Verification items for the finished model (mm, model axes). Face numbers are marked on the shaded views. A direction names the side the tool comes from. Coordinates: 2 decimals unless noted, no trailing zeros. Write each loop counter-clockwise with the first axis right and the second up, starting at its lowest first coordinate (ties: lowest second). Pieces come first, ordered by that corner, then holes. Notation, with made-up numbers: M -14.75,83 L -1.75,83 A27 cw -1.75,121 Z; hole C 47,84 d11. An arc over 180 degrees is marked long. One line per item, written item: value.
```python
from build123d import *

# Parameters (mm, degrees)
BOSS_EXTRUDE1_DEPTH = 70.612
SKETCH2_R           = 2.2
CUT_EXTRUDE1_DEPTH  = 83.799422419
SKETCH3_W           = 8.255
SKETCH3_H           = 31.401404102
CUT_EXTRUDE2_DEPTH  = 83.799422419
BOSS_EXTRUDE3_DEPTH = 2.54
CUT_EXTRUDE6_DEPTH  = 2.54
SKETCH9_W           = 51.816
SKETCH9_H           = 2.54
CUT_EXTRUDE7_DEPTH  = 2.54
FILLET1_R           = 1.27
FILLET2_R           = 1.27
SKETCH11_W          = 16.51
SKETCH11_H          = 8.89
CUT_EXTRUDE8_DEPTH  = 2.54


with BuildPart() as part:
    # Sketch1 → Boss-Extrude1 (new body)
    with BuildSketch(Plane.XY):
        Polygon((25.908, 25.4), (-25.908, 25.4), (-25.908, 0), (-36.703, 0), (-36.703, 5.08), (-28.448, 5.08), (-28.448, 27.94), (28.448, 27.94), (28.448, 5.08), (36.703, 5.08), (36.703, 0), (25.908, 0), align=None)
    extrude(amount=BOSS_EXTRUDE1_DEPTH)

    # Sketch2 → Cut-Extrude1 (cut, through all)
    with BuildSketch(Plane(origin=(0, 5.08, 0), x_dir=(1, 0, 0), z_dir=(0, 1, 0))):
        with Locations(Location((-32.5755, -6.35, 0), (0, 0, 270))):
            Circle(SKETCH2_R)
        with Locations(Location((-32.5755, -29.21, 0), (0, 0, 270))):
            Circle(SKETCH2_R)
    cut_extrude1 = extrude(amount=-CUT_EXTRUDE1_DEPTH, mode=Mode.SUBTRACT)

    # Mirror1: Cut-Extrude1 across plane
    add(cut_extrude1.mirror(Plane(origin=(0, 0, 0), x_dir=(0, 0, 1), z_dir=(1, 0, 0))), mode=Mode.SUBTRACT)

    # Sketch3 → Cut-Extrude2 (cut, through all)
    with BuildSketch(Plane(origin=(0, 5.08, 0), x_dir=(1, 0, 0), z_dir=(0, 1, 0))):
        with Locations((-32.5755, -54.911297949)):
            Rectangle(SKETCH3_W, SKETCH3_H)
        with Locations((32.5755, -54.911297949)):
            Rectangle(SKETCH3_W, SKETCH3_H)
    extrude(amount=-CUT_EXTRUDE2_DEPTH, mode=Mode.SUBTRACT)

    # Sketch6 → Boss-Extrude3 (add)
    with BuildSketch(Plane(origin=(0, 0, 0), x_dir=(-1, 0, 0), z_dir=(0, 0, -1))):
        Polygon((-25.908, 0), (25.908, 0), (36.703, 0), (36.703, 5.08), (28.448, 5.08), (28.448, 27.94), (-28.448, 27.94), (-28.448, 5.08), (-36.703, 5.08), (-36.703, 0), align=None)
    extrude(amount=-BOSS_EXTRUDE3_DEPTH)

    # Sketch8 → Cut-Extrude6 (cut)
    with BuildSketch(Plane(origin=(0, 0, 0), x_dir=(-1, 0, 0), z_dir=(0, 0, -1))):
        with BuildLine():
            Line((-15.875, 0), (15.875, 0))
            ThreePointArc((15.875, 0), (0, 7.635884934), (-15.875, 0))
        make_face()
    extrude(amount=-CUT_EXTRUDE6_DEPTH, mode=Mode.SUBTRACT)

    # Sketch9 → Cut-Extrude7 (cut)
    with BuildSketch(Plane(origin=(0, 0, 0), x_dir=(-1, 0, 0), z_dir=(0, 0, -1))):
        with Locations((0, 1.27)):
            Rectangle(SKETCH9_W, SKETCH9_H)
    extrude(amount=-CUT_EXTRUDE7_DEPTH, mode=Mode.SUBTRACT)

    # Fillet1
    fillet1_edges = [part.edges().sort_by_distance(p)[0] for p in [
        (-25.908, 0, 35.306),
        (-28.448, 27.94, 35.306),
        (28.448, 27.94, 35.306),
        (25.908, 0, 35.306),
        (-36.703, 0, 19.605297949),
        (-36.703, 5.08, 19.605297949),
        (-28.448, 5.08, 19.605297949),
        (28.448, 5.08, 19.605297949),
        (36.703, 5.08, 19.605297949),
        (36.703, 0, 19.605297949),
        (-28.448, 0, 54.911297949),
        (28.448, 0, 54.911297949),
    ]]
    fillet(fillet1_edges, radius=FILLET1_R - 0.0001)  # a hair under: the kernel refuses the full size

    # Fillet2
    fillet2_edges = [part.edges().sort_by_distance(p)[0] for p in [
        (-25.908, 2.54, 1.27),
        (25.908, 2.54, 1.27),
    ]]
    fillet(fillet2_edges, radius=FILLET2_R)

    # Sketch11 → Cut-Extrude8 (cut)
    with BuildSketch(Plane(origin=(0, 0, 0), x_dir=(-1, 0, 0), z_dir=(0, 0, -1))):
        with Locations((10.16, 18.034)):
            Rectangle(SKETCH11_W, SKETCH11_H)
    extrude(amount=-CUT_EXTRUDE8_DEPTH, mode=Mode.SUBTRACT)


solid = part.part
```
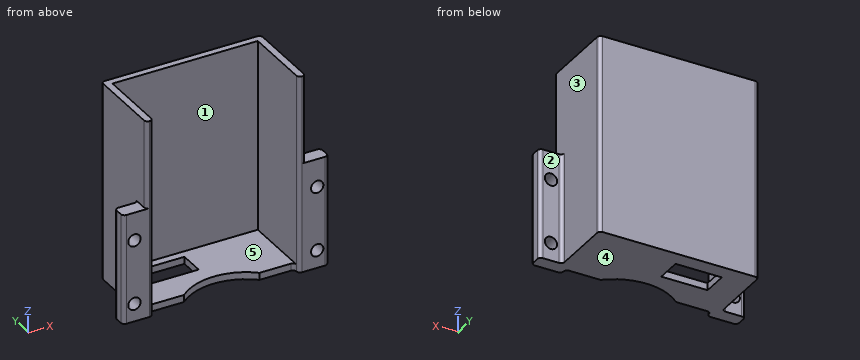
Item 1: Go/stop test with flat-tipped pins: P1, Ø2, axis at y = 19, z = 2, coming from the -X side; P2, Ø3, axis at y = 19.5, z = 1.5, coming from the +X side; P3, Ø10, axis at y = 9.5, z = 20, coming from the -X side. Record where each tip stops, or that it passes through.
The answers:
P1: stops at x = -28.45
P2: stops at x = 28.45
P3: stops at x = -36.5
Item 2: Cross-section at C-C, the plane z = 16. Enter the section's corners in (x, y).
The answers:
outline: M -36.7,1.27 A1.27 ccw -35.43,0 L -27.18,0 A1.27 ccw -25.91,1.27 L -25.91,25.4 L 25.91,25.4 L 25.91,1.27 A1.27 ccw 27.18,0 L 35.43,0 A1.27 ccw 36.7,1.27 L 36.7,3.81 A1.27 ccw 35.43,5.08 L 29.72,5.08 A1.27 cw 28.45,6.35 L 28.45,26.67 A1.27 ccw 27.18,27.94 L -27.18,27.94 A1.27 ccw -28.45,26.67 L -28.45,6.35 A1.27 cw -29.72,5.08 L -35.43,5.08 A1.27 ccw -36.7,3.81 Z
Item 3: Scan lines: line 1 (X direction, y = 1.8, z = 6.35); line 2 (X direction, y = 15.75, z = 26); line 3 (Y direction, x = -16.5, z = 19.5). Record each from-to range of solid material in increasing order.
The answers:
line 1: x = -36.7 to -34.78, -30.38 to -25.91, 25.91 to 30.38, 34.78 to 36.7
line 2: x = -28.45 to -25.91, 25.91 to 28.45
line 3: y = 25.4 to 27.94
Item 4: Draft check along X on the marked faces 1, 2 and 3. Enter one of: released by +X, released by -X, zero draft, split by the parting line, or undercut.
The answers:
face 1: undercut
face 2: zero draft
face 3: released by +X
Item 5: Cross-section at A-A, the plane y = 16.5. Enter the section's corners in (x, z) (3 decimals).
The answers:
outline: M -28.448,0 L -18.415,0 L -18.415,2.54 L -25.908,2.54 L -25.908,70.612 L -28.448,70.612 Z; M -1.905,0 L 28.448,0 L 28.448,70.612 L 25.908,70.612 L 25.908,2.54 L -1.905,2.54 Z
Item 6: Cross-section at B-B, the plane z = 29.21. Give the number of separate pieces and of enclosed holes in the cut face, and give its area (3 significant figures).
The answers:
separate pieces: 3
enclosed holes: 0
area: 311 mm²
Item 7: Access from +Z, -Z, +X, -X, +Y, -Y to the whole of each face (thin tool, end or side, straight path). Record for the marked faces 4 and 5.
The answers:
face 4: -Z, +X, -X, +Y, -Y
face 5: +Z, -Y
Item 8: Cross-section at D-D, the plane x = -31.5. Enter the section's corners in (y, z), and give its area (3 significant figures).
The answers:
outline: M 0,0 L 5.08,0 L 5.08,4.43 L 0,4.43 Z; M 0,8.27 L 5.08,8.27 L 5.08,27.29 L 0,27.29 Z; M 0,31.13 L 5.08,31.13 L 5.08,39.21 L 0,39.21 Z
area: 160 mm²
